```python
from build123d import *

# Parameters (mm, degrees)
SKETCH1_W               = 16
SKETCH1_H               = 5
BOSS_EXTRUDE1_DEPTH     = 30
BOSS_EXTRUDE2_DEPTH     = 14
CUT_EXTRUDE1_DEPTH      = 33.691742077
CUT_EXTRUDE1_DEPTH_BACK = 33.691742077
BOSS_EXTRUDE3_START     = 30
SKETCH1_3_W             = 16
SKETCH1_3_H             = 5
BOSS_EXTRUDE3_DEPTH     = 10
SKETCH5_W               = 16
SKETCH5_H               = 0.5
BOSS_EXTRUDE4_DEPTH     = 40


with BuildPart() as part:
    # Sketch1 → Boss-Extrude1 (new body)
    with BuildSketch(Plane(origin=(0, 0, 0), x_dir=(1, 0, 0), z_dir=(0, 1, 0))):
        Rectangle(SKETCH1_W, SKETCH1_H)
        with BuildLine():
            Line((2.5, -9.25), (2.5, -2.5))
            Line((2.5, -2.5), (-2.5, -2.5))
            Line((-2.5, -2.5), (-2.5, -9.25))
            ThreePointArc((-2.5, -9.25), (0, -9.160600109), (2.5, -9.25))
        make_face()
    extrude(amount=BOSS_EXTRUDE1_DEPTH)

    # Sketch2 → Boss-Extrude2 (add)
    with BuildSketch(Plane(origin=(0, 0, 0), x_dir=(1, 0, 0), z_dir=(0, 1, 0))):
        with BuildLine():
            ThreePointArc((32.691742077, -31.660600109), (0, -9.160600109), (-32.691742077, -31.660600109))
            Line((-32.691742077, -31.660600109), (-24.213890642, -31.660600109))
            ThreePointArc((-24.213890642, -31.660600109), (0, -16.910600109), (24.213890642, -31.660600109))
            Line((24.213890642, -31.660600109), (32.691742077, -31.660600109))
        make_face()
    extrude(amount=BOSS_EXTRUDE2_DEPTH)

    # Sketch3 → Cut-Extrude1 (cut, two sides)
    with BuildSketch(Plane(origin=(0, 0, 0), x_dir=(0, 0, -1), z_dir=(1, 0, 0))) as cut_extrude1_sk:
        Polygon((-9.25, 14), (-31.660600109, 14), (-31.660600109, 0), align=None)
    extrude(amount=CUT_EXTRUDE1_DEPTH, mode=Mode.SUBTRACT)
    extrude(cut_extrude1_sk.sketch, amount=-CUT_EXTRUDE1_DEPTH_BACK, mode=Mode.SUBTRACT)

    # Sketch1_3 → Boss-Extrude3 (add)
    with BuildSketch(Plane(origin=(0, 0, 0), x_dir=(1, 0, 0), z_dir=(0, 1, 0)).offset(BOSS_EXTRUDE3_START)):
        Rectangle(SKETCH1_3_W, SKETCH1_3_H)
    extrude(amount=BOSS_EXTRUDE3_DEPTH)

    # Sketch5 → Boss-Extrude4 (add)
    with BuildSketch(Plane(origin=(0, 40, 0), x_dir=(1, 0, 0), z_dir=(0, 1, 0))):
        with Locations((0, -2.75)):
            Rectangle(SKETCH5_W, SKETCH5_H)
    extrude(amount=-BOSS_EXTRUDE4_DEPTH)


solid = part.part
```
Work out the finished part from the listing and answer in its coordinate system (mm). A direction names the side the tool comes from. Give positions to 0.01 mm unless a question says otherwise; leave off trailing zeros. Loops run counter-clockwise (first coordinate to the right, second up) from the corner with the lowest first, then second, coordinate; pieces in that order, holes last. Notation, with made-up numbers: (52.25, -6.75) -> (63.25, -6.75) arc R23 cw to (63.25, 15.25) -> close; hole circle Ø1 at (60.25, 63). An arc over 180 degrees is marked (long way). Put each result on its own line as item: value. Start each with the question number.
Item 1: Which of the six approach directions +Z, -Z, +X, -X, +Y, -Y give full straight-line access (tool end or side, diameter ignored) to faces 5 (the face through (0, 30, 6)), 6 (the face through (-2.5, 15, 6)), 7 (the face through (-8, 20, 0))?
Item 2: Each of these flat-tipped pins is pushed along its axis until it touches: P1, Ø6, axis at y = 24.5, z = 1, coming from the -X side; P2, Ø3, axis at y = 12.5, z = 5.5, coming from the -X side; P3, Ø5, axis at x = 10, z = 17, coming from the +Y side; P4, Ø3, axis at x = -10.5, y = 36, coming from the +Z side. Where does it stop, or does it pass through?
Item 3: The part is cut by section C-C (x = -6.5). Give the vertices of the cut face in (y, z).
Item 4: The part is cut by section B-B (y = 20.5). Give the vertices of the cut face in (x, z).
Item 5: The part is cut by section D-D (z = 6). Give the vertices of the cut face in (x, y).
Item 6: The mould has two halves that part along Z. Classify faces 1 (the face through (0, 20, -2.5)), 2 (the face through (-0.458, 10.013, 15.632)), 3 (the face through (2.5, 15, 6)), 4 (the face through (8, 20, 0)): released by +Z, released by -Z, zero draft, split by the parting line, or undercut.
Item 7: The part is cut by section A-A (z = 24.5). Give the vertices of the cut face in (x, y).
Item 8: Find the intervals of material crossed by L1, parallel to X at y = 4, z = 2.5; L2, parallel to Y at x = -0.5, z = 4; L3, parallel to X at y = 27, z = 3.5, in increasing order. Write a range as [from, to].
Answers below:
1. face 5: +Z, +X, -X, +Y
1. face 6: -X, +Y, -Y
1. face 7: -Z, -X, +Y, -Y
2. P1: x = -8
2. P2: x = -2.5
2. P3: y = 10.72
2. P4: through
3. outline: (0, -2.5) -> (40, -2.5) -> (40, 3) -> (0, 3) -> close; (0, 9.77) -> (13.68, 9.77) -> (8.72, 17.7) -> (0, 17.7) -> close
4. outline: (-8, -2.5) -> (8, -2.5) -> (8, 3) -> (2.5, 3) -> (2.5, 9.25) arc R35 cw to (-2.5, 9.25) -> (-2.5, 3) -> (-8, 3) -> close
5. outline: (-2.5, 0) -> (2.5, 0) -> (2.5, 30) -> (-2.5, 30) -> close
6. face 1: released by -Z
6. face 2: released by +Z
6. face 3: undercut
6. face 4: zero draft
7. outline: (-28.96, 0) -> (-18.87, 0) -> (-18.87, 4.47) -> (-28.96, 4.47) -> close; (18.87, 0) -> (28.96, 0) -> (28.96, 4.47) -> (18.87, 4.47) -> close
8. L1: [-8, 8]
8. L2: [0, 30]
8. L3: [-2.5, 2.5]
